Geometry: final body of the model. Coordinates: model frame, mm. A direction names the side the tool comes from. Round coordinates to 2 decimals unless told otherwise and drop trailing zeros. Loops run counter-clockwise (first coordinate to the right, second up) from the corner with the lowest first, then second, coordinate; pieces in that order, holes last. Notation, with made-up numbers: (21, 21.25) -> (29, 21.25) arc R21 ccw to (29, 50.25) -> close; hole circle Ø2 at (72, 12). An arc over 180 degrees is marked (long way). Answer in a Markdown table with one row per item.
```python
from build123d import *

# Parameters (mm, degrees)
SKETCH1_W                       = 80
SKETCH1_H                       = 98.8
BOSS_EXTRUDE1_DEPTH             = 3
BOSS_EXTRUDE2_DEPTH             = 3
CHAMFER2_SIZE                   = 2
FILLET1_R                       = 2
SKETCH4_W                       = 11
SKETCH4_H                       = 3
BOSS_EXTRUDE3_DEPTH             = 4.1
SKETCH6_W                       = 11
SKETCH6_H                       = 32.1
BOSS_EXTRUDE4_DEPTH             = 3
CHAMFER3_SIZE                   = 2
F_3_0MM_DOWEL_HOLE1_D           = 3.2
F_3_0MM_DOWEL_HOLE1_CSINK_D     = 3.25
F_3_0MM_DOWEL_HOLE1_CSINK_ANGLE = 90
F_3_0MM_DOWEL_HOLE2_D           = 3
F_3_0MM_DOWEL_HOLE2_DEPTH       = 20
F_3_0MM_DOWEL_HOLE2_CSINK_D     = 3.05
F_3_0MM_DOWEL_HOLE2_CSINK_ANGLE = 90
F_3_0MM_DOWEL_HOLE2_TIP         = 0.901290929


with BuildPart() as part:
    # Sketch1 → Boss-Extrude1 (new body)
    with BuildSketch(Plane(origin=(0, 0, 0), x_dir=(1, 0, 0), z_dir=(0, 1, 0))):
        Rectangle(SKETCH1_W, SKETCH1_H)
    extrude(amount=BOSS_EXTRUDE1_DEPTH)

    # Sketch3 → Boss-Extrude2 (add)
    with BuildSketch(Plane.XY.offset(49.4)):
        Polygon((-40, 0), (-40, 3), (40, 3), (40, 0), (5.5, -52), (-5.5, -52), align=None)
    boss_extrude2 = extrude(amount=BOSS_EXTRUDE2_DEPTH)

    # Mirror1: Boss-Extrude2 across plane
    add(boss_extrude2.mirror(Plane.XY))

    # Chamfer2
    chamfer2_edges = [part.edges().sort_by_distance(p)[0] for p in [
        (0, 0, 49.4),
        (0, 0, -49.4),
    ]]
    chamfer(chamfer2_edges, length=CHAMFER2_SIZE)

    # Fillet1
    fillet1_edges = [part.edges().sort_by_distance(p)[0] for p in [
        (40, 1.5, 52.4),
        (-40, 1.5, 52.4),
        (-40, 1.5, -52.4),
        (40, 1.5, -52.4),
    ]]
    fillet(fillet1_edges, radius=FILLET1_R)

    # Sketch4 → Boss-Extrude3 (add)
    with BuildSketch(Plane(origin=(0, 0, 49.4), x_dir=(-1, 0, 0), z_dir=(0, 0, -1))):
        with Locations((0, -21.4)):
            Rectangle(SKETCH4_W, SKETCH4_H)
    boss_extrude3 = extrude(amount=BOSS_EXTRUDE3_DEPTH)

    # Sketch6 → Boss-Extrude4 (add)
    with BuildSketch(Plane(origin=(0, 0, 45.3), x_dir=(-1, 0, 0), z_dir=(0, 0, -1))):
        with Locations((0, -35.95)):
            Rectangle(SKETCH6_W, SKETCH6_H)
    boss_extrude4 = extrude(amount=BOSS_EXTRUDE4_DEPTH)

    # Mirror4: Boss-Extrude3, Boss-Extrude4 across plane
    add(boss_extrude3.mirror(Plane.XY))
    add(boss_extrude4.mirror(Plane.XY))

    # Chamfer3
    chamfer3_edges = [part.edges().sort_by_distance(p)[0] for p in [
        (0, -19.9, 49.4),
        (0, -19.9, -49.4),
    ]]
    chamfer(chamfer3_edges, length=CHAMFER3_SIZE)

    # Ø3.0mm Dowel Hole1 (through all)
    with Locations(Plane.XY.offset(52.4)):
        with Locations((0, -47), (0, -38), (0, -29)):
            CounterSinkHole(F_3_0MM_DOWEL_HOLE1_D / 2, F_3_0MM_DOWEL_HOLE1_CSINK_D / 2, counter_sink_angle=F_3_0MM_DOWEL_HOLE1_CSINK_ANGLE)

    # Ø3.0mm Dowel Hole2
    with Locations(Plane(origin=(0, 3, 0), x_dir=(1, 0, 0), z_dir=(0, 1, 0))):
        with Locations((-24.35, 25), (-24.35, -25)):
            CounterSinkHole(F_3_0MM_DOWEL_HOLE2_D / 2, F_3_0MM_DOWEL_HOLE2_CSINK_D / 2, depth=F_3_0MM_DOWEL_HOLE2_DEPTH, counter_sink_angle=F_3_0MM_DOWEL_HOLE2_CSINK_ANGLE)
            with Locations((0, 0, -(F_3_0MM_DOWEL_HOLE2_DEPTH + F_3_0MM_DOWEL_HOLE2_TIP / 2))):  # 118° drill point
                Cone(0, F_3_0MM_DOWEL_HOLE2_D / 2, F_3_0MM_DOWEL_HOLE2_TIP, mode=Mode.SUBTRACT)


solid = part.part
```
Item 1: First-contact query: P1, Ø3, axis at x = 0, y = -38, coming from the +Z side; P2, Ø5.5, axis at y = -28, z = -44, coming from the +X side; P3, Ø24, axis at x = 18.5, z = 2.5, coming from the -Y side; P4, Ø8, axis at y = -40.5, z = 47.5, coming from the +X side. Flat tips, straight axial feed; report the tip coordinate or a pass-through.
Ans:
| item | result |
|---|---|
| P1 | through |
| P2 | x = 5.5 |
| P3 | y = 0 |
| P4 | x = 15.47 |
Item 2: Mould query, pull axis X, two halves, no side actions, for faces 4 (the flat face through (0, -52, 44)), 5 (the cylindrical face through (-0.74, -39.42, 43.78)), 6 (the flat face through (22.99, -25.64, 50.98)). Classes: released by +X, released by -X, zero draft, split by the parting line, or undercut.
Ans:
| item | result |
|---|---|
| face 4 | zero draft |
| face 5 | undercut |
| face 6 | released by +X |
Item 3: Section query B-B, the plane y = -12. Output: boundary loops of the cut face in (x, z), and give its area (3 significant figures).
Ans:
| item | result |
|---|---|
| outline | (-32.04, -52.4) -> (32.04, -52.4) -> (32.04, -49.4) -> (-32.04, -49.4) -> close; (-32.04, 49.4) -> (32.04, 49.4) -> (32.04, 52.4) -> (-32.04, 52.4) -> close |
| area | 384 mm2 |
Item 4: Set-up query: faces 1 (the flat face through (3, -37, -45.3)), 2 (the flat face through (5.5, -35, 44)), 3 (the flat face through (0, -19.9, -45)). Return all of +Z, -Z, +X, -X, +Y, -Y with unobstructed straight access to the full face (end or side cutting, diameter ignored); none if empty.
Ans:
| item | result |
|---|---|
| face 1 | +X, -X, -Y |
| face 2 | +X, -Y |
| face 3 | +X, -X |
Item 5: Ray query, L1, parallel to Y at x = 0, z = 43.5; L2, parallel to Y at x = 0, z = -51.1; L3, parallel to Z at x = 14, y = -34.5. Return the intervals inside material, ascending.
Ans:
| item | result |
|---|---|
| L1 | -52 to -48.6, -45.4 to -39.6, -36.4 to -30.6, -27.4 to -19.9, 0 to 3 |
| L2 | -52 to -48.6, -45.4 to -39.6, -36.4 to -30.6, -27.4 to 3 |
| L3 | -52.4 to -49.4, 49.4 to 52.4 |
Item 6: Section query C-C, the plane x = 3. Output: boundary loops of the cut face in (y, z).
Ans:
| item | result |
|---|---|
| outline | (-52, -52.4) -> (3, -52.4) -> (3, 52.4) -> (-52, 52.4) -> (-52, 49.4) -> (-22.9, 49.4) -> (-22.9, 45.3) -> (-52, 45.3) -> (-52, 42.3) -> (-19.9, 42.3) -> (-19.9, 47.4) -> (-17.9, 49.4) -> (-2, 49.4) -> (0, 47.4) -> (0, -47.4) -> (-2, -49.4) -> (-17.9, -49.4) -> (-19.9, -47.4) -> (-19.9, -42.3) -> (-52, -42.3) -> (-52, -45.3) -> (-22.9, -45.3) -> (-22.9, -49.4) -> (-52, -49.4) -> close |
Item 7: Section query A-A, the plane z = -25. Output: boundary loops of the cut face in (x, y) (3 decimals), and give its area (3 significant figures).
Ans:
| item | result |
|---|---|
| outline | (-40, 0) -> (-25.85, 0) -> (-25.85, 2.975) -> (-25.875, 3) -> (-40, 3) -> close; (-22.85, 0) -> (40, 0) -> (40, 3) -> (-22.825, 3) -> (-22.85, 2.975) -> close |
| area | 231 mm2 |
Item 8: Section query D-D, the plane y = -38. State how many separate pieces and enclosed holes the cut face has, and give its area (3 significant figures).
Ans:
| item | result |
|---|---|
| separate pieces | 8 |
| enclosed holes | 0 |
| area | 205 mm2 |
